Solid Edge part; units mm, degrees
sketch "Sketch1" plane through (0, 0, 0) normal (0, -1, 0) x (1, 0, 0)
  line L0 (50, 0) -> (50, 60)
  line L1 (50, 60) -> (0, 60)
  line L2 (0, 60) -> (0, 0)
  line L3 (0, 0) -> (50, 0)
extrude "Protrusion1" add sketch "Sketch1" against normal blind 100
hole "Bohrung_1" at (30, 80, 60) direction (0, 0, -1) diameter 11 end up to next
hole "Hole1" at (30, 20, 60) direction (0, 0, -1) diameter 11 end up to next
sketch "Sketch2" plane through (50, 50, 30) normal (1, 0, 0) x (0, 1, 0)
  circle A0 centre (0, 0) radius 10
extrude "Extrusionsausprägung_2" add sketch "Sketch2" along normal blind 160
Check sheet for the modelled part. Datum: model origin and axes. Units: mm. A direction names the side the tool comes from. Round coordinates to 2 decimals unless told otherwise and drop trailing zeros. Loops run counter-clockwise (first coordinate to the right, second up) from the corner with the lowest first, then second, coordinate; pieces in that order, holes last. Notation, with made-up numbers: (71, 39.25) -> (121, 39.25) arc R33 ccw to (121, 69.25) -> close; hole circle Ø9 at (66.5, 8). An arc over 180 degrees is marked (long way). Put each result on its own line as item: value. Start each with the question number.
1. Gauge pin test, flat ends, axial feed: pin 1 (14.5 mm diameter, centred on x = 30, y = 20, fed in from +Z); pin 2 (12 mm diameter, centred on x = 59.5, y = 61.5, fed in from +Z); pin 3 (10 mm diameter, centred on y = 37, z = 21, fed in from +X). Record the tip position at first contact, or that the pin passes through.
2. Section check D-D (y = 50). Enter the section's corners in (x, z).
3. Access from +Z, -Z, +X, -X, +Y, -Y to the whole of each face (thin tool, end or side, straight path). Record for faces 5 (the face through (129, 42, 36)), 6 (the face through (25, 49, 60)).
4. Draft check along X on faces 1 (the face through (35.453, 20.716, 30.42)), 2 (the face through (25, 100, 30)), 3 (the face through (30.242, 85.495, 30.42)), 4 (the face through (210, 50, 30)). Enter one of: +X half, -X half, draft (parallel to the pull), parting line (faces both ways), or undercut.
5. Section check C-C (z = 30). Enter the section's corners in (x, y).
6. Section check A-A (y = 20). Enter the section's corners in (x, z).
7. Scan lines: probe 1 along Y at (x, z) = (30, 45.5); probe 2 along X at (y, z) = (20, 12.5); probe 3 along X at (y, z) = (61, 55.5). Record each from-to range of solid material in increasing order.
8. Section check B-B (x = 30). Enter the section's corners in (y, z).
Findings:
1. pin 1: stops at z = 60
1. pin 2: stops at z = 38.35
1. pin 3: stops at x = 50
2. outline: (0, 0) -> (50, 0) -> (50, 20) -> (210, 20) -> (210, 40) -> (50, 40) -> (50, 60) -> (0, 60) -> close
3. face 5: +X
3. face 6: +Z, +X, -X, +Y, -Y
4. face 1: undercut
4. face 2: draft
4. face 3: undercut
4. face 4: +X half
5. outline: (0, 0) -> (50, 0) -> (50, 40) -> (210, 40) -> (210, 60) -> (50, 60) -> (50, 100) -> (0, 100) -> close; hole circle Ø11 at (30, 20); hole circle Ø11 at (30, 80)
6. outline: (0, 0) -> (24.5, 0) -> (24.5, 60) -> (0, 60) -> close; (35.5, 0) -> (50, 0) -> (50, 60) -> (35.5, 60) -> close
7. probe 1: y = 0 to 14.5, 25.5 to 74.5, 85.5 to 100
7. probe 2: x = 0 to 24.5, 35.5 to 50
7. probe 3: x = 0 to 50
8. outline: (0, 0) -> (14.5, 0) -> (14.5, 60) -> (0, 60) -> close; (25.5, 0) -> (74.5, 0) -> (74.5, 60) -> (25.5, 60) -> close; (85.5, 0) -> (100, 0) -> (100, 60) -> (85.5, 60) -> close
